```python
from build123d import *

# Parameters (mm, degrees)
SKETCH2_W               = 63.52
SKETCH2_H               = 30.59
BOSS_EXTRUDE1_DEPTH     = 7
SKETCH3_W               = 3
SKETCH3_H               = 30.59
BOSS_EXTRUDE2_DEPTH     = 40
FILLET2_R               = 3
SKETCH4_R               = 1.25
CUT_EXTRUDE2_DEPTH      = 70
CUT_EXTRUDE4_DEPTH      = 6
CUT_EXTRUDE4_DEPTH_BACK = 20
SKETCH7_R               = 1.25
SKETCH7_R_2             = 1.249999994
SKETCH11_W              = 4
SKETCH11_H              = 3
CUT_EXTRUDE5_DEPTH      = 80


with BuildPart() as part:
    # Sketch2 → Boss-Extrude1 (new body)
    with BuildSketch(Plane(origin=(0, 0, 0), x_dir=(1, 0, 0), z_dir=(0, 1, 0))):
        with Locations((-20.26308022, 14.924105874)):
            Rectangle(SKETCH2_W, SKETCH2_H)
    extrude(amount=BOSS_EXTRUDE1_DEPTH)

    # Sketch3 → Boss-Extrude2 (add)
    with BuildSketch(Plane(origin=(0, 7, 0), x_dir=(1, 0, 0), z_dir=(0, 1, 0))):
        with Locations((-50.52308022, 14.924105874)):
            Rectangle(SKETCH3_W, SKETCH3_H)
        with Locations((9.99691978, 14.924105874)):
            Rectangle(SKETCH3_W, SKETCH3_H)
    extrude(amount=BOSS_EXTRUDE2_DEPTH)

    # Fillet2
    fillet2_edges = [part.edges().sort_by_distance(p)[0] for p in [
        (11.49691978, 0, -14.924105874),
        (-52.02308022, 0, -14.924105874),
    ]]
    fillet(fillet2_edges, radius=FILLET2_R)

    # Sketch4 → Cut-Extrude2 (cut)
    with BuildSketch(Plane.ZY.offset(52.02308022)):
        with BuildLine():
            ThreePointArc((-25.359340899, 37.664418298), (-21.924948962, 44.325483759), (-14.924105874, 47))
            Line((-14.924105874, 47), (-30.219105874, 47))
            Line((-30.219105874, 47), (-30.219105874, 3))
            Line((-30.219105874, 3), (-25.359340899, 37.664418298))
        make_face()
        with BuildLine():
            Line((0.370894126, 47), (-14.924105874, 47))
            ThreePointArc((-14.924105874, 47), (-7.923262787, 44.325483759), (-4.488870849, 37.664418298))
            Line((-4.488870849, 37.664418298), (0.370894126, 3))
            Line((0.370894126, 3), (0.370894126, 47))
        make_face()
        with Locations((-7.424105874, 36.5)):
            Circle(SKETCH4_R)
        with Locations((-7.424105874, 40)):
            Circle(SKETCH4_R)
        with Locations((-7.424105874, 33)):
            Circle(SKETCH4_R)
        with Locations((-14.924105874, 29)):
            Circle(SKETCH4_R)
        with Locations((-11.424105874, 29)):
            Circle(SKETCH4_R)
        with Locations((-18.424105874, 29)):
            Circle(SKETCH4_R)
        with Locations((-22.424105874, 36.5)):
            Circle(SKETCH4_R)
        with Locations((-22.424105874, 40)):
            Circle(SKETCH4_R)
        with Locations((-22.424105874, 33)):
            Circle(SKETCH4_R)
        with Locations((-11.424105874, 44)):
            Circle(SKETCH4_R)
        with Locations((-18.424105874, 44)):
            Circle(SKETCH4_R)
        with Locations((-14.924105874, 44)):
            Circle(SKETCH4_R)
    extrude(amount=-CUT_EXTRUDE2_DEPTH, mode=Mode.SUBTRACT)

    # Sketch7 → Cut-Extrude4 (cut, two sides: drawn at the far end of the back side and taken through both)
    with BuildSketch(Plane(origin=(0, 7, 0), x_dir=(1, 0, 0), z_dir=(0, 1, 0)).offset(-CUT_EXTRUDE4_DEPTH_BACK)):
        with Locations(Location((-11.073080223, 11.041478624, 0), (0, 0, 270))):
            Circle(SKETCH7_R)
        with Locations(Location((-11.073080223, 22.304987192, 0), (0, 0, 270))):
            Circle(SKETCH7_R)
        with Locations(Location((-29.454080223, 11.041478624, 0), (0, 0, 270))):
            Circle(SKETCH7_R_2)
        with Locations(Location((-29.454080223, 22.304987192, 0), (0, 0, 270))):
            Circle(SKETCH7_R)
    extrude(amount=CUT_EXTRUDE4_DEPTH + CUT_EXTRUDE4_DEPTH_BACK, mode=Mode.SUBTRACT)

    # Sketch11 → Cut-Extrude5 (cut)
    with BuildSketch(Plane.ZY.offset(52.02308022)):
        with Locations((-16.924105874, 11.5)):
            Rectangle(SKETCH11_W, SKETCH11_H)
        with Locations((-12.924105874, 11.5)):
            Rectangle(SKETCH11_W, SKETCH11_H)
    extrude(amount=-CUT_EXTRUDE5_DEPTH, mode=Mode.SUBTRACT)


solid = part.part
```
Source: CAD feature listing. Evaluate the final solid. Frame: model axes, mm. A direction names the side the tool comes from. Coordinates: 2 decimals unless noted, no trailing zeros. Order: outer loops, then holes, each group sorted by start corner. A loop starts at its lowest first (then second) coordinate and runs counter-clockwise, first axis right, second up. Notation, with made-up numbers: (35.25, 61) - (72.25, 61) arc R11 ccw to (72.25, 74) - close; hole circle Ø1 at (60.5, 38). An arc over 180 degrees is marked (long way). One line per item, written item: value.
1) Reachability of faces 1 (the face through (-51, 11, -10.924)), 2 (the face through (-10.228, 3.451, -11.963)) from +Z, -Z, +X, -X, +Y, -Y: full face, straight path, thin tool, end or side. Return the list, or none.
Computed values:
face 1: +X, -X
face 2: +Y, -Y
2) Contact query for flat-ended pins moving along their axis: pin 1 (6 mm diameter, centred on x = 2.5, y = 29, fed in from +Z); pin 2 (3 mm diameter, centred on x = -45, z = -4.5, fed in from +Y); pin 3 (1.5 mm diameter, centred on x = -7, y = 7, fed in from -Z); pin 4 (3.5 mm diameter, centred on x = -51, z = -15, fed in from -Y). Output: stop coordinate, or through.
Computed values:
pin 1: passes through
pin 2: stops at y = 7
pin 3: stops at z = -29.76
pin 4: stops at y = 0.01
3) Cut plane D-D on x = -20. Output: boundary loops of the cut face in (y, z).
Computed values:
outline: (0, -30.22) - (3, -30.22) - (7, -29.66) - (7, -0.19) - (3, 0.37) - (0, 0.37) - close
4) Cut plane B-B on y = 12. Output: boundary loops of the cut face in (x, z), plus the area to 3 significant figures.
Computed values:
outline: (-52.02, -28.96) - (-49.02, -28.96) - (-49.02, -18.92) - (-52.02, -18.92) - close; (-52.02, -10.92) - (-49.02, -10.92) - (-49.02, -0.89) - (-52.02, -0.89) - close; (8.5, -28.96) - (11.5, -28.96) - (11.5, -18.92) - (8.5, -18.92) - close; (8.5, -10.92) - (11.5, -10.92) - (11.5, -0.89) - (8.5, -0.89) - close
area: 120 mm^2
5) Ray query, line 1 (X direction, y = 19.5, z = -22); line 2 (Y direction, x = -25.5, z = -20.5); line 3 (Z direction, x = -27, y = 4). Return the intervals inside material, ascending. Write a range as [from, to].
Computed values:
line 1: x = [-52.02, -49.02], [8.5, 11.5]
line 2: y = [0, 7]
line 3: z = [-30.08, 0.23]
6) Cut plane C-C on y = 29. State how many separate pieces and enclosed holes the cut face has, plus the area to 3 significant figures.
Computed values:
separate pieces: 8
enclosed holes: 0
area: 94.8 mm^2
7) Cut plane A-A on y = 36.5. Output: boundary loops of the cut face in (x, z), plus the area to 3 significant figures.
Computed values:
outline: (-52.02, -25.52) - (-49.02, -25.52) - (-49.02, -23.67) - (-52.02, -23.67) - close; (-52.02, -21.17) - (-49.02, -21.17) - (-49.02, -8.67) - (-52.02, -8.67) - close; (-52.02, -6.17) - (-49.02, -6.17) - (-49.02, -4.33) - (-52.02, -4.33) - close; (8.5, -25.52) - (11.5, -25.52) - (11.5, -23.67) - (8.5, -23.67) - close; (8.5, -21.17) - (11.5, -21.17) - (11.5, -8.67) - (8.5, -8.67) - close; (8.5, -6.17) - (11.5, -6.17) - (11.5, -4.33) - (8.5, -4.33) - close
area: 97.2 mm^2
8) Mould query, pull axis X, two halves, no side actions, for faces 3 (the face through (-10.7, 3.45, -21.11)), 4 (the face through (-51.168, 0.902, -15.138)), 5 (the face through (-50.54, 35.28, -22.7)). Classes: released by +X, released by -X, zero draft, split by the parting line, or undercut.
Computed values:
face 3: undercut
face 4: released by -X
face 5: zero draft
